Part model, mm, in its own coordinate system. A direction names the side the tool comes from. Round coordinates to 2 decimals unless told otherwise and drop trailing zeros. Loops run counter-clockwise (first coordinate to the right, second up) from the corner with the lowest first, then second, coordinate; pieces in that order, holes last.
(1) Flat gauge pins, fed straight in: pin 1 (2 mm diameter, centred on x = -1.5, y = -2, fed in from +Z); pin 2 (3 mm diameter, centred on x = -10.5, y = -0.5, fed in from -Z); pin 3 (2 mm diameter, centred on x = 12, z = 2.5, fed in from +Y); pin 4 (2.5 mm diameter, centred on x = 5.66, y = 5.66, fed in from +Z). Where does each tip first touch, or does it go through?
(2) Cut at A-A on z = 31.5. List the corners of the cut face in (x, y), then the cut area to 3 significant figures.
(3) Probe probe 1 along Y at (x, z) = (-0.25, 8); probe 2 along Y at (x, z) = (1.75, 18.5); probe 3 along X at (y, z) = (-0.25, 33). List the from-to ranges inside material, lowest first.
(4) Mould opens along X. For faces 6 (the face through (3, 9, 19.5)), 7 (the face through (-3.994, 12.411, 23.162)), 8 (the face through (-3.095, -2.373, 27.106)) say: +X half, -X half, draft (parallel to the pull), parting line (faces both ways), or undercut.
(5) Tool access for faces 1 (the face through (3, -9, 19.5)), 2 (the face through (0, -6.9, 2)), 3 (the face through (1.5, 0.07, -0.9)), 4 (the face through (-5.182, 8.927, 21.718)), 5 (the face through (-0.59, -2.68, 33.34)): list every direction of +Z, -Z, +X, -X, +Y, -Y with a clear straight run to the whole face (end or side of a thin tool).
from build123d import *

# Parameters (mm, degrees)
SKETCH1_R           = 13.9
BOSS_EXTRUDE1_DEPTH = 24
FILLET1_R           = 0.5
CUT_EXTRUDE1_DEPTH  = 4
CUT_EXTRUDE2_DEPTH  = 4
SKETCH4_R           = 4
BOSS_EXTRUDE2_DEPTH = 0.1
SKETCH5_R           = 3
BOSS_EXTRUDE3_DEPTH = 0.5
SKETCH6_R           = 1.5
BOSS_EXTRUDE4_DEPTH = 0.6
SKETCH7_R           = 1.5
CUT_EXTRUDE3_DEPTH  = 4
CHAMFER1_SIZE       = 1.7
CUT_EXTRUDE4_START  = -4.5
CUT_EXTRUDE4_DEPTH  = 4.5
SKETCH9_R           = 3.9
BOSS_EXTRUDE5_DEPTH = 6.3
CUT_EXTRUDE5_START  = -4.3
CUT_EXTRUDE5_DEPTH  = 4.3
SKETCH10_R          = 2.9
BOSS_EXTRUDE6_DEPTH = 6.8
SKETCH16_W          = 0.5
SKETCH16_H          = 0.5
SKETCH16_H_2        = 0.2


# Read off the part's stored shape, not the designer's step: #12-24 Machine Threads Stud1
with BuildPart() as part:
    # Sketch1 → Boss-Extrude1 (new body)
    with BuildSketch(Plane.XY):
        Circle(SKETCH1_R)
    extrude(amount=BOSS_EXTRUDE1_DEPTH)

    # Fillet1
    fillet1_edges = [part.edges().sort_by_distance(p)[0] for p in [
        (-13.9, 0, 0),
    ]]
    fillet(fillet1_edges, radius=FILLET1_R)

    # Sketch2 → Cut-Extrude1 (cut)
    with BuildSketch(Plane(origin=(0, 0, 0), x_dir=(-1, 0, 0), z_dir=(0, 0, -1))):
        with BuildLine():
            Line((-13.572398462, 3), (-9.572398462, 3))
            ThreePointArc((-9.572398462, 3), (-6.572398365, 0), (-9.572398462, -3))
            Line((-9.572398462, -3), (-13.572398462, -3))
            ThreePointArc((-13.572398462, -3), (-13.9, 0), (-13.572398462, 3))
        make_face()
        with BuildLine():
            Line((3, 13.572398462), (3, 9.572398462))
            ThreePointArc((3, 9.572398462), (0, 6.572398365), (-3, 9.572398462))
            Line((-3, 9.572398462), (-3, 13.572398462))
            ThreePointArc((-3, 13.572398462), (0, 13.9), (3, 13.572398462))
        make_face()
        with BuildLine():
            Line((13.572398462, -3), (9.572398462, -3))
            ThreePointArc((9.572398462, -3), (6.572398365, 0), (9.572398462, 3))
            Line((9.572398462, 3), (13.572398462, 3))
            ThreePointArc((13.572398462, 3), (13.9, 0), (13.572398462, -3))
        make_face()
    extrude(amount=-CUT_EXTRUDE1_DEPTH, mode=Mode.SUBTRACT)

    # Sketch3 → Cut-Extrude2 (cut)
    with BuildSketch(Plane(origin=(0, 0, 0), x_dir=(-1, 0, 0), z_dir=(0, 0, -1))):
        with BuildLine():
            Line((-5, -12.969579793), (-2.5, -8.384373134))
            ThreePointArc((-2.5, -8.384373134), (0, -6.9), (2.5, -8.384373134))
            Line((2.5, -8.384373134), (5, -12.969579793))
            ThreePointArc((5, -12.969579793), (0, -13.9), (-5, -12.969579793))
        make_face()
    extrude(amount=-CUT_EXTRUDE2_DEPTH, mode=Mode.SUBTRACT)

    # Sketch4 → Boss-Extrude2 (add)
    with BuildSketch(Plane(origin=(0, 0, 0), x_dir=(-1, 0, 0), z_dir=(0, 0, -1))):
        with Locations(Location((0, 0, 0), (0, 0, 180))):
            Circle(SKETCH4_R)
    extrude(amount=BOSS_EXTRUDE2_DEPTH)

    # Sketch5 → Boss-Extrude3 (add)
    with BuildSketch(Plane(origin=(0, 0, -0.1), x_dir=(-1, 0, 0), z_dir=(0, 0, -1))):
        Circle(SKETCH5_R)
    extrude(amount=BOSS_EXTRUDE3_DEPTH)

    # Sketch6 → Boss-Extrude4 (add)
    with BuildSketch(Plane(origin=(0, 0, -0.6), x_dir=(-1, 0, 0), z_dir=(0, 0, -1))):
        Circle(SKETCH6_R)
    extrude(amount=BOSS_EXTRUDE4_DEPTH)

    # Sketch7 → Cut-Extrude3 (cut)
    with BuildSketch(Plane(origin=(0, 0, 0), x_dir=(-1, 0, 0), z_dir=(0, 0, -1))):
        with Locations((-5.656854249, 5.656854249)):
            Circle(SKETCH7_R)
        with Locations((6.717514421, 6.717514421)):
            Circle(SKETCH7_R)
        with Locations((5.656854249, -5.656854249)):
            Circle(SKETCH7_R)
        with Locations((-6.717514421, -6.717514421)):
            Circle(SKETCH7_R)
    extrude(amount=-CUT_EXTRUDE3_DEPTH, mode=Mode.SUBTRACT)

    # Chamfer1
    chamfer1_edges = [part.edges().sort_by_distance(p)[0] for p in [
        (-13.9, 0, 24),
    ]]
    chamfer(chamfer1_edges, length=CHAMFER1_SIZE)

    # Sketch8 → Cut-Extrude4 (cut)
    with BuildSketch(Plane.XY.offset(24).offset(CUT_EXTRUDE4_START)):
        with BuildLine():
            Line((12.585706178, 5.9), (6.380828907, 2.5))
            ThreePointArc((6.380828907, 2.5), (4.9, 0), (6.380828907, -2.5))
            Line((6.380828907, -2.5), (12.585706178, -5.9))
            ThreePointArc((12.585706178, -5.9), (13.9, 0), (12.585706178, 5.9))
        make_face()
        with BuildLine():
            Line((9.500430541, -10.146517606), (4.349425861, -5.295986426))
            ThreePointArc((4.349425861, -5.295986426), (1.514183272, -4.66017693), (-0.40585672, -6.841071398))
            Line((-0.40585672, -6.841071398), (-1.722036351, -13.79291814))
            ThreePointArc((-1.722036351, -13.79291814), (4.295336222, -13.219685577), (9.500430541, -10.146517606))
        make_face()
        with BuildLine():
            Line((-6.714117196, -12.170892748), (-3.692735894, -5.773099615))
            ThreePointArc((-3.692735894, -5.773099615), (-3.964183272, -2.880147736), (-6.631662155, -1.728014643))
            Line((-6.631662155, -1.728014643), (-13.649983173, -2.624492214))
            ThreePointArc((-13.649983173, -2.624492214), (-11.245336222, -8.170215007), (-6.714117196, -12.170892748))
        make_face()
        with BuildLine():
            Line((-13.649983173, 2.624492214), (-6.631662155, 1.728014643))
            ThreePointArc((-6.631662155, 1.728014643), (-3.964183272, 2.880147736), (-3.692735894, 5.773099615))
            Line((-3.692735894, 5.773099615), (-6.714117196, 12.170892748))
            ThreePointArc((-6.714117196, 12.170892748), (-11.245336222, 8.170215007), (-13.649983173, 2.624492214))
        make_face()
        with BuildLine():
            Line((-1.722036351, 13.79291814), (-0.40585672, 6.841071398))
            ThreePointArc((-0.40585672, 6.841071398), (1.514183272, 4.66017693), (4.349425861, 5.295986426))
            Line((4.349425861, 5.295986426), (9.500430541, 10.146517606))
            ThreePointArc((9.500430541, 10.146517606), (4.295336222, 13.219685577), (-1.722036351, 13.79291814))
        make_face()
    extrude(amount=CUT_EXTRUDE4_DEPTH, mode=Mode.SUBTRACT)

    # Sketch9 → Boss-Extrude5 (add)
    with BuildSketch(Plane.XY.offset(24)):
        Circle(SKETCH9_R)
    extrude(amount=BOSS_EXTRUDE5_DEPTH)

    # Sketch11 → Cut-Extrude5 (cut)
    with BuildSketch(Plane.XY.offset(30.3).offset(CUT_EXTRUDE5_START)):
        with BuildLine():
            Line((3.375, 1.954322133), (3.375, -1.954322133))
            ThreePointArc((3.375, -1.954322133), (3.9, 0), (3.375, 1.954322133))
        make_face()
        with BuildLine():
            Line((-3.375, 1.954322133), (-3.375, -1.954322133))
            ThreePointArc((-3.375, -1.954322133), (-3.9, 0), (-3.375, 1.954322133))
        make_face()
    extrude(amount=CUT_EXTRUDE5_DEPTH, mode=Mode.SUBTRACT)

    # Sketch10 → Boss-Extrude6 (add)
    with BuildSketch(Plane.XY.offset(30.3)):
        Circle(SKETCH10_R)
    extrude(amount=BOSS_EXTRUDE6_DEPTH)

    # #12-24 Machine Threads Stud1 outline → #12-24 Machine Threads Stud1 (revolve, cut)
    with BuildSketch(Plane.XZ):
        Polygon((2.7432, 36.47008), (2.7432, 30.3), (2.9, 30.3), (2.9, 37.1), (2.11328, 37.1), align=None)
    revolve(axis=Axis((0, 0, 0), (0, 0, 1)), mode=Mode.SUBTRACT)

    # Sketch16 → Cut-Revolve1 (revolve, cut)
    with BuildSketch(Plane(origin=(0, 0, 0), x_dir=(1, 0, 0), z_dir=(0, 1, 0))):
        with Locations((-13.65, -5.25)):
            Rectangle(SKETCH16_W, SKETCH16_H)
        with Locations((13.65, -18.7)):
            Rectangle(SKETCH16_W, SKETCH16_H_2)
    revolve(axis=Axis((0, 0, -7.765685178), (0, 0, 1)), mode=Mode.SUBTRACT)


solid = part.part
Final values:
1. pin 1: stops at z = 37.1
1. pin 2: stops at z = 4
1. pin 3: stops at y = 8.5
1. pin 4: stops at z = 24
2. outline: circle Ø5.49 at (0, 0)
2. area: 23.6 mm2
3. probe 1: y = -13.9 to 13.9
3. probe 2: y = -13.79 to 13.79
3. probe 3: x = -2.73 to 2.73
4. face 6: undercut
4. face 7: -X half
4. face 8: parting line
5. face 1: +Z, -Y
5. face 2: -Z, -Y
5. face 3: -Z
5. face 4: +Z, -X
5. face 5: +Z
